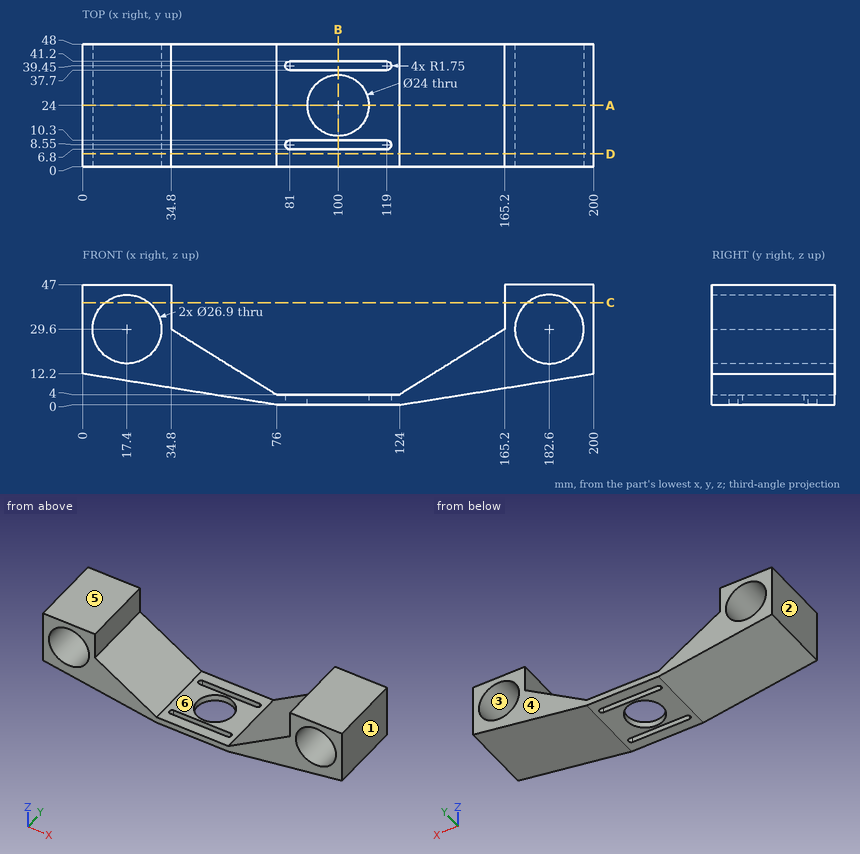
The figure shows three views and two pictorial views of one solid part (mm, origin at its lowest corner). Answer the questions. A direction names the side the tool comes from. Round coordinates to 2 decimals unless told otherwise and drop trailing zeros. Write each loop counter-clockwise with the first axis right and the second up, starting at its lowest first coordinate (ties: lowest second). Pieces come first, ordered by that corner, then holes. Notation, with made-up numbers: M 0,67 L 49,67 A21 ccw 49,100 Z; hole C -11.75,20 d3. An arc over 180 degrees is marked long. Use a Markdown table: item, result.
1) Flat-ended cylindrical pins translate along their axes: pin 1 (1.2 mm diameter, centred on x = 91, z = 3, fed in from -Y); pin 2 (1 mm diameter, centred on x = 121.5, y = 19, fed in from +Z); pin 3 (4 mm diameter, centred on x = 173.5, y = 15, fed in from -Z) (3 decimals); pin 4 (1.5 mm diameter, centred on x = 31, y = 34.5, fed in from -Z). Find the tip coordinate at first contact, or state that the pin passes through.
Taken from the geometry:
| item | result |
|---|---|
| pin 1 | stops at y = 0 |
| pin 2 | stops at z = 4 |
| pin 3 | stops at z = 7.625 |
| pin 4 | stops at z = 7.1 |
2) The part is cut by section A-A on y = 24. Give the vertices of the cut face in (x, z), plus the area to 3 significant figures.
Taken from the geometry:
| item | result |
|---|---|
| outline | M 0,12.2 L 76,0 L 88,0 L 88,4 L 76,4 L 34.8,29.6 L 34.8,47 L 0,47 Z; M 112,0 L 124,0 L 200,12.2 L 200,47 L 165.2,47 L 165.2,29.6 L 124,4 L 112,4 Z; hole C 17.4,29.6 d26.9; hole C 182.6,29.6 d26.9 |
| area | 2,690 mm2 |
3) The part is cut by section D-D on y = 5. Give the vertices of the cut face in (x, z).
Taken from the geometry:
| item | result |
|---|---|
| outline | M 0,12.2 L 76,0 L 124,0 L 200,12.2 L 200,47 L 165.2,47 L 165.2,29.6 L 124,4 L 76,4 L 34.8,29.6 L 34.8,47 L 0,47 Z; hole C 17.4,29.6 d26.9; hole C 182.6,29.6 d26.9 |
4) Which of the six approach directions +Z, -Z, +X, -X, +Y, -Y give full straight-line access (tool end or side, diameter ignored) to the marked faces 5 and 6?
Taken from the geometry:
| item | result |
|---|---|
| face 5 | +Z, +X, -X, +Y, -Y |
| face 6 | +Z, +Y, -Y |
5) Determine the mould class of the marked faces 1, 2, 3 and 4 for opening direction X: pulls with the +X half, pulls with the -X half, needs draft (parallel to the pull), parting line crosses it, or undercut.
Taken from the geometry:
| item | result |
|---|---|
| face 1 | pulls with the +X half |
| face 2 | pulls with the -X half |
| face 3 | undercut |
| face 4 | needs draft |
6) The part is cut by section C-C on z = 40. Give the vertices of the cut face in (x, y).
Taken from the geometry:
| item | result |
|---|---|
| outline | M 0,0 L 8.87,0 L 8.87,48 L 0,48 Z; M 25.93,0 L 34.8,0 L 34.8,48 L 25.93,48 Z; M 165.2,0 L 174.07,0 L 174.07,48 L 165.2,48 Z; M 191.13,0 L 200,0 L 200,48 L 191.13,48 Z |
7) The part is cut by section B-B on x = 100. Give the vertices of the cut face in (y, z), plus the area to 3 significant figures.
Taken from the geometry:
| item | result |
|---|---|
| outline | M 0,0 L 6.8,0 L 6.8,4 L 0,4 Z; M 10.3,0 L 12,0 L 12,4 L 10.3,4 Z; M 36,0 L 37.7,0 L 37.7,4 L 36,4 Z; M 41.2,0 L 48,0 L 48,4 L 41.2,4 Z |
| area | 68.0 mm2 |
8) Consider line 1 (X direction, y = 35, z = 29.6); line 2 (X direction, y = 27.5, z = 20.5); line 3 (X direction, y = 14, z = 45). Determine where each line is inside the solid, lowest interval first. Write a range as [from, to].
Taken from the geometry:
| item | result |
|---|---|
| line 1 | x = [0, 3.95], [30.85, 34.8], [165.2, 169.15], [196.05, 200] |
| line 2 | x = [0, 7.5], [27.3, 49.45], [150.55, 172.7], [192.5, 200] |
| line 3 | x = [0, 34.8], [165.2, 200] |
